Here's how the part is built. I have some questions about the finished solid (model axes, mm). Round coordinates to 2 decimals unless told otherwise and drop trailing zeros. Order: outer loops, then holes, each group sorted by start corner. A loop starts at its lowest first (then second) coordinate and runs counter-clockwise, first axis right, second up. Notation, with made-up numbers: (85, 35.5) -> (129, 35.5) arc R23 ccw to (129, 70.5) -> close; hole circle Ø8 at (36, 89). An arc over 180 degrees is marked (long way). Answer in a Markdown table with one row per item.
```python
from build123d import *

# Parameters (mm, degrees)
SKETCH_1_R              = 3
EXTRUDE_1_DEPTH         = 1.5
SHEET_START             = -1.5
SHEET_METAL_1_OUTLINE_R = 3
SHEET_METAL_1_DEPTH     = 1.5


# Read off the part's stored shape, not the designer's step: Преобразовать-Твердое тело1
with BuildPart() as part:
    # Sketch 1 → Бобышка-Вытянуть1 (new body)
    with BuildSketch(Plane.XY):
        with BuildLine():
            Line((389.31902002, 22), (75, 22))
            Line((75, 22), (75, -153))
            ThreePointArc((75, -153), (0, -228), (-75, -153))
            Line((-75, -153), (-75, 22))
            Line((-75, 22), (-389.31902002, 22))
            ThreePointArc((-389.31902002, 22), (-397.979274058, 17), (-397.979274058, 7))
            Line((-397.979274058, 7), (-376.299038106, -30.551270189))
            Line((-376.299038106, -30.551270189), (-392.320508076, -39.801270189))
            Line((-392.320508076, -39.801270189), (-382.320508076, -57.121778265))
            Line((-382.320508076, -57.121778265), (-366.299038106, -47.871778265))
            Line((-366.299038106, -47.871778265), (-241.299038106, -264.378129211))
            Line((-241.299038106, -264.378129211), (-257.320508076, -273.628129211))
            Line((-257.320508076, -273.628129211), (-247.320508076, -290.948637287))
            Line((-247.320508076, -290.948637287), (-231.299038106, -281.698637287))
            Line((-231.299038106, -281.698637287), (-203.75277675, -329.410161514))
            ThreePointArc((-203.75277675, -329.410161514), (-200.092522712, -333.070415552), (-195.092522712, -334.410161514))
            Line((-195.092522712, -334.410161514), (-149.133974596, -334.410161514))
            Line((-149.133974596, -334.410161514), (-149.133974596, -352.910161514))
            Line((-149.133974596, -352.910161514), (-129.133974596, -352.910161514))
            Line((-129.133974596, -352.910161514), (-129.133974596, -334.410161514))
            Line((-129.133974596, -334.410161514), (129.133974596, -334.410161514))
            Line((129.133974596, -334.410161514), (129.133974596, -352.910161514))
            Line((129.133974596, -352.910161514), (149.133974596, -352.910161514))
            Line((149.133974596, -352.910161514), (149.133974596, -334.410161514))
            Line((149.133974596, -334.410161514), (195.092522712, -334.410161514))
            ThreePointArc((195.092522712, -334.410161514), (200.092522712, -333.070415552), (203.75277675, -329.410161514))
            Line((203.75277675, -329.410161514), (231.299038106, -281.698637287))
            Line((231.299038106, -281.698637287), (247.320508076, -290.948637287))
            Line((247.320508076, -290.948637287), (257.320508076, -273.628129211))
            Line((257.320508076, -273.628129211), (241.299038106, -264.378129211))
            Line((241.299038106, -264.378129211), (366.299038106, -47.871778265))
            Line((366.299038106, -47.871778265), (382.320508076, -57.121778265))
            Line((382.320508076, -57.121778265), (392.320508076, -39.801270189))
            Line((392.320508076, -39.801270189), (376.299038106, -30.551270189))
            Line((376.299038106, -30.551270189), (397.979274058, 7))
            ThreePointArc((397.979274058, 7), (397.979274058, 17), (389.31902002, 22))
        make_face()
        with Locations((244.309773091, -277.663383249)):
            Circle(SKETCH_1_R, mode=Mode.SUBTRACT)
        with Locations((379.309773091, -43.836524227)):
            Circle(SKETCH_1_R, mode=Mode.SUBTRACT)
        with Locations((139.133974596, -343.660161514)):
            Circle(SKETCH_1_R, mode=Mode.SUBTRACT)
        with Locations((-139.133974596, -343.660161514)):
            Circle(SKETCH_1_R, mode=Mode.SUBTRACT)
        with Locations((-244.309773091, -277.663383249)):
            Circle(SKETCH_1_R, mode=Mode.SUBTRACT)
        with Locations((-379.309773091, -43.836524227)):
            Circle(SKETCH_1_R, mode=Mode.SUBTRACT)
        with Locations((300, 10)):
            Circle(SKETCH_1_R, mode=Mode.SUBTRACT)
        with Locations((-300, 10)):
            Circle(SKETCH_1_R, mode=Mode.SUBTRACT)
    extrude(amount=EXTRUDE_1_DEPTH)

    # Sheet Metal 1 outline → Sheet Metal 1 (add)
    with BuildSketch(Plane.XY.offset(SHEET_START)):
        with BuildLine():
            Line((-149.133974596, -334.410161514), (-149.133974596, -352.910161514))
            Line((-149.133974596, -352.910161514), (-129.133974596, -352.910161514))
            Line((-129.133974596, -352.910161514), (-129.133974596, -334.410161514))
            Line((-129.133974596, -334.410161514), (129.133974596, -334.410161514))
            Line((129.133974596, -334.410161514), (129.133974596, -352.910161514))
            Line((129.133974596, -352.910161514), (149.133974596, -352.910161514))
            Line((149.133974596, -352.910161514), (149.133974596, -334.410161514))
            Line((149.133974596, -334.410161514), (195.092522712, -334.410161514))
            ThreePointArc((195.092522712, -334.410161514), (200.092522712, -333.070415552), (203.75277675, -329.410161514))
            Line((203.75277675, -329.410161514), (231.299038106, -281.698637287))
            Line((231.299038106, -281.698637287), (247.320508076, -290.948637287))
            Line((247.320508076, -290.948637287), (257.320508076, -273.628129211))
            Line((257.320508076, -273.628129211), (241.299038106, -264.378129211))
            Line((241.299038106, -264.378129211), (366.299038106, -47.871778265))
            Line((366.299038106, -47.871778265), (382.320508076, -57.121778265))
            Line((382.320508076, -57.121778265), (392.320508076, -39.801270189))
            Line((392.320508076, -39.801270189), (376.299038106, -30.551270189))
            Line((376.299038106, -30.551270189), (397.979274058, 7))
            ThreePointArc((397.979274058, 7), (397.979274058, 17), (389.31902002, 22))
            Line((389.31902002, 22), (75, 22))
            Line((75, 22), (75, -153))
            ThreePointArc((75, -153), (0, -228), (-75, -153))
            Line((-75, -153), (-75, 22))
            Line((-75, 22), (-389.31902002, 22))
            ThreePointArc((-389.31902002, 22), (-397.979274058, 17), (-397.979274058, 7))
            Line((-397.979274058, 7), (-376.299038106, -30.551270189))
            Line((-376.299038106, -30.551270189), (-392.320508076, -39.801270189))
            Line((-392.320508076, -39.801270189), (-382.320508076, -57.121778265))
            Line((-382.320508076, -57.121778265), (-366.299038106, -47.871778265))
            Line((-366.299038106, -47.871778265), (-241.299038106, -264.378129211))
            Line((-241.299038106, -264.378129211), (-257.320508076, -273.628129211))
            Line((-257.320508076, -273.628129211), (-247.320508076, -290.948637287))
            Line((-247.320508076, -290.948637287), (-231.299038106, -281.698637287))
            Line((-231.299038106, -281.698637287), (-203.75277675, -329.410161514))
            ThreePointArc((-203.75277675, -329.410161514), (-200.092522712, -333.070415552), (-195.092522712, -334.410161514))
            Line((-195.092522712, -334.410161514), (-149.133974596, -334.410161514))
        make_face()
        with Locations((-244.309773091, -277.663383249)):
            Circle(SHEET_METAL_1_OUTLINE_R, mode=Mode.SUBTRACT)
        with Locations((-139.133974596, -343.660161514)):
            Circle(SHEET_METAL_1_OUTLINE_R, mode=Mode.SUBTRACT)
        with Locations((139.133974596, -343.660161514)):
            Circle(SHEET_METAL_1_OUTLINE_R, mode=Mode.SUBTRACT)
        with Locations((244.309773091, -277.663383249)):
            Circle(SHEET_METAL_1_OUTLINE_R, mode=Mode.SUBTRACT)
        with Locations((-379.309773091, -43.836524227)):
            Circle(SHEET_METAL_1_OUTLINE_R, mode=Mode.SUBTRACT)
        with Locations((-300, 10)):
            Circle(SHEET_METAL_1_OUTLINE_R, mode=Mode.SUBTRACT)
        with Locations((379.309773091, -43.836524227)):
            Circle(SHEET_METAL_1_OUTLINE_R, mode=Mode.SUBTRACT)
        with Locations((300, 10)):
            Circle(SHEET_METAL_1_OUTLINE_R, mode=Mode.SUBTRACT)
    extrude(amount=SHEET_METAL_1_DEPTH)


solid = part.part
```
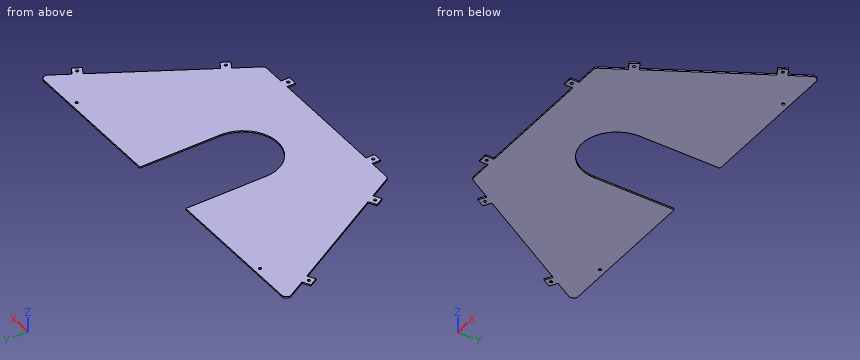
1. Suppose I cut it at D-D on x = 327. Write out the boundary of the cut face in (y, z), then the cut area to 3 significant figures.
Numbers:
| item | result |
|---|---|
| outline | (-115.94, -1.5) -> (22, -1.5) -> (22, 1.5) -> (-115.94, 1.5) -> close |
| area | 414 mm2 |
2. For pin 1 Ø1.5 at (y, z) = (-103.5, 0.5) entering from +X; pin 2 Ø1 at (x, z) = (44.5, -1) entering from -Y; pin 3 Ø1 at (y, z) = (-23.5, 0) entering from +X, each with a flat end and sliding along its axis, tell me the tip position at first contact or that it passes through.
Numbers:
| item | result |
|---|---|
| pin 1 | stops at x = 334.62 |
| pin 2 | stops at y = -334.41 |
| pin 3 | stops at x = 380.66 |
3. Please list where these lines run through material, in increasing order: line 1 along X through (y, z) = (-279.5, -0.2); line 2 along X through (y, z) = (-285, 1.4); line 3 along X through (y, z) = (-38, 0.25).
Numbers:
| item | result |
|---|---|
| line 1 | x = -253.93 to -246.68, -241.94 to 241.94, 246.68 to 253.93 |
| line 2 | x = -250.75 to -237.02, -229.39 to 229.39, 237.02 to 250.75 |
| line 3 | x = -389.2 to -75, 75 to 389.2 |
4. Suppose I cut it at A-A on y = -207. Write out the boundary of the cut face in (x, z), then the cut area to 3 significant figures.
Numbers:
| item | result |
|---|---|
| outline | (-274.43, -1.5) -> (-52.05, -1.5) -> (-52.05, 1.5) -> (-274.43, 1.5) -> close; (52.05, -1.5) -> (274.43, -1.5) -> (274.43, 1.5) -> (52.05, 1.5) -> close |
| area | 1,330 mm2 |
5. Suppose I cut it at B-B on x = 0. Write out the boundary of the cut face in (y, z).
Numbers:
| item | result |
|---|---|
| outline | (-334.41, -1.5) -> (-228, -1.5) -> (-228, 1.5) -> (-334.41, 1.5) -> close |
6. Suppose I cut it at C-C on z = -0.05. State how many separate pieces and enclosed holes the cut face has, then the cut area to 3 significant figures.
Numbers:
| item | result |
|---|---|
| separate pieces | 1 |
| enclosed holes | 8 |
| area | 183,000 mm2 |
